Verification items for the finished model (mm, model axes). Face numbers are marked on the shaded views. A direction names the side the tool comes from. Coordinates: 2 decimals unless noted, no trailing zeros. Order: outer loops, then holes, each group sorted by start corner. A loop starts at its lowest first (then second) coordinate and runs counter-clockwise, first axis right, second up.
Q1. Cross-section at C-C, the plane y = 6.75. Record the boundary of the cut face in (x, z) (3 decimals).
Q2. Cross-section at B-B, the plane x = 6.35. Record the boundary of the cut face in (y, z).
Q3. Thickness scan on line 1 (Y direction, x = -1.27, z = 0.75); line 2 (X direction, y = 5.5, z = 2.5); line 3 (Z direction, x = -6.75, y = 10.25). Record the ranges inside material, lowest first.
Q4. Cross-section at A-A, the plane y = -3.16. Record the boundary of the cut face in (x, z).
Q5. Set-up check for the marked faces 1 and 2: record each of +Z, -Z, +X, -X, +Y, -Y from which the full face is reachable in a straight line by a thin tool's end or side.
Q6. Depth check by flat-ended pin: P1, Ø2, axis at x = 3.5, z = 3, coming from the +Y side; P2, Ø0.8, axis at x = 2, z = 3.5, coming from the +Y side; P3, Ø2, axis at x = 1, z = 3, coming from the -Y side; P4, Ø0.5, axis at y = 7, z = 2.5, coming from the -X side. Enter the tip coordinate at first touch or a pass-through.
Q7. Cross-section at D-D, the plane z = 1.25. Count the separate pieces of the cut face and the enclosed holes in it, and give its area (3 significant figures).
from build123d import *

# Parameters (mm, degrees)
SKETCH_W        = 17.7
SKETCH_H        = 21.4
PAD_DEPTH       = 1.65
SKETCH001_W     = 9
SKETCH001_H     = 7.4
PAD001_DEPTH    = 3.35
SKETCH002_R     = 0.5
POCKET_DEPTH    = 1.651
FILLET_R        = 1.675
POCKET001_DEPTH = 2
POCKET002_DEPTH = 4.5
POCKET003_DEPTH = 0.35


with BuildPart() as part:
    # Sketch → Pad (new body)
    with BuildSketch(Plane.XY):
        Rectangle(SKETCH_W, SKETCH_H)
    extrude(amount=PAD_DEPTH)

    # Sketch001 (on Face6 of Pad) → Pad001 (join)
    with BuildSketch(Plane.XY.offset(1.65)):
        with Locations((0, 7.3)):
            Rectangle(SKETCH001_W, SKETCH001_H)
    extrude(amount=PAD001_DEPTH)

    # Sketch002 (on Face5 of Pad001) → Pocket (cut, through all)
    with BuildSketch(Plane.XY.offset(1.65)):
        with Locations((-6.35, -3.16)):
            Circle(SKETCH002_R)
        with Locations((-3.81, -3.16)):
            Circle(SKETCH002_R)
        with Locations((-1.27, -3.16)):
            Circle(SKETCH002_R)
        with Locations((1.27, -3.16)):
            Circle(SKETCH002_R)
        with Locations((3.81, -3.16)):
            Circle(SKETCH002_R)
        with Locations((6.35, -3.16)):
            Circle(SKETCH002_R)
        with Locations((-6.35, -5.7)):
            Circle(SKETCH002_R)
        with Locations((-3.81, -5.7)):
            Circle(SKETCH002_R)
        with Locations((-1.27, -5.7)):
            Circle(SKETCH002_R)
        with Locations((1.27, -5.7)):
            Circle(SKETCH002_R)
        with Locations((3.81, -5.7)):
            Circle(SKETCH002_R)
        with Locations((6.35, -5.7)):
            Circle(SKETCH002_R)
    extrude(amount=-POCKET_DEPTH, mode=Mode.SUBTRACT)

    # Fillet
    fillet_edges = [part.edges().sort_by_distance(p)[0] for p in [
        (-4.5, 7.3, 5),
        (4.5, 7.3, 5),
    ]]
    fillet(fillet_edges, radius=FILLET_R)

    # Sketch003 (on Face5 of Fillet) → Pocket001 (cut)
    with BuildSketch(Plane(origin=(0, 11, 0), x_dir=(-1, 0, 0), z_dir=(0, 1, 0))):
        with BuildLine():
            ThreePointArc((-4.5, 3.325), (-4.009404, 2.140596), (-2.825, 1.65))
            Line((-2.825, 1.65), (-4.5, 1.65))
            Line((-4.5, 3.325), (-4.5, 1.65))
        make_face()
        with BuildLine():
            ThreePointArc((2.825, 1.65), (4.009404, 2.140596), (4.5, 3.325))
            Line((4.5, 3.325), (4.5, 1.65))
            Line((2.825, 1.65), (4.5, 1.65))
        make_face()
    extrude(amount=-POCKET001_DEPTH, mode=Mode.SUBTRACT)

    # Sketch004 (on Face6 of Pocket001) → Pocket002 (cut)
    with BuildSketch(Plane(origin=(0, 11, 0), x_dir=(-1, 0, 0), z_dir=(0, 1, 0))):
        with BuildLine():
            ThreePointArc((-2.825, 4.7), (-4.2, 3.325), (-2.825, 1.95))
            Line((-2.825, 1.95), (2.825, 1.95))
            ThreePointArc((2.825, 1.95), (4.2, 3.325), (2.825, 4.7))
            Line((2.825, 4.7), (-2.825, 4.7))
        make_face()
        with BuildLine():
            ThreePointArc((-2.825, 3.65), (-3.15, 3.325), (-2.825, 3))
            Line((-2.825, 3), (2.825, 3))
            ThreePointArc((2.825, 3), (3.15, 3.325), (2.825, 3.65))
            Line((2.825, 3.65), (-2.825, 3.65))
        make_face(mode=Mode.SUBTRACT)
    extrude(amount=-POCKET002_DEPTH, mode=Mode.SUBTRACT)

    # Pocket002 Face38 → Pocket003 (cut)
    with BuildSketch(Plane(origin=(0, 11, 3.325), x_dir=(1, 0, 0), z_dir=(0, 1, 0))):
        with BuildLine():
            Line((-2.825, -0.325), (2.825, -0.325))
            ThreePointArc((2.825, -0.325), (3.15, 0), (2.825, 0.325))
            Line((2.825, 0.325), (-2.825, 0.325))
            ThreePointArc((-2.825, 0.325), (-3.15, 0), (-2.825, -0.325))
        make_face()
    extrude(amount=-POCKET003_DEPTH, mode=Mode.SUBTRACT)


solid = part.part
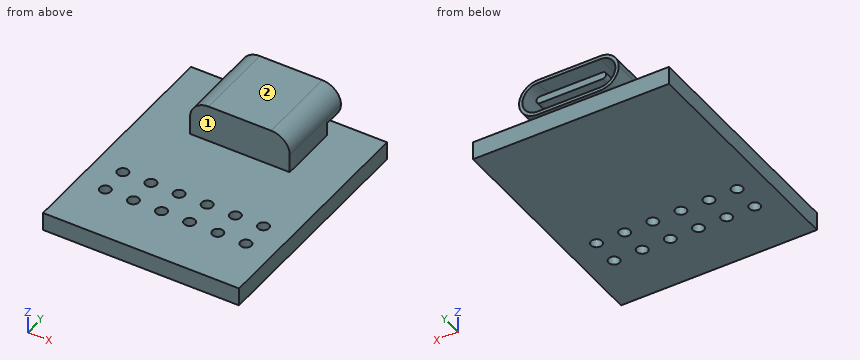
Check values:
1. outline: (-8.85, 0) - (8.85, 0) - (8.85, 1.65) - (4.5, 1.65) - (4.5, 3.325) arc R1.675 ccw to (2.825, 5) - (-2.825, 5) arc R1.675 ccw to (-4.5, 3.325) - (-4.5, 1.65) - (-8.85, 1.65) - close; (-2.825, 3) - (2.825, 3) arc R0.325 ccw to (2.825, 3.65) - (-2.825, 3.65) arc R0.325 ccw to start; hole (-2.825, 1.95) - (2.825, 1.95) arc R1.375 ccw to (2.825, 4.7) - (-2.825, 4.7) arc R1.375 ccw to start
2. outline: (-10.7, 0) - (-6.2, 0) - (-6.2, 1.65) - (-10.7, 1.65) - close; (-5.2, 0) - (-3.66, 0) - (-3.66, 1.65) - (-5.2, 1.65) - close; (-2.66, 0) - (10.7, 0) - (10.7, 1.65) - (-2.66, 1.65) - close
3. line 1: y = -10.7 to -6.2, -5.2 to -3.66, -2.66 to 10.7
3. line 2: x = -4.5 to 4.5
3. line 3: z = 0 to 1.65
4. outline: (-8.85, 0) - (-6.85, 0) - (-6.85, 1.65) - (-8.85, 1.65) - close; (-5.85, 0) - (-4.31, 0) - (-4.31, 1.65) - (-5.85, 1.65) - close; (-3.31, 0) - (-1.77, 0) - (-1.77, 1.65) - (-3.31, 1.65) - close; (-0.77, 0) - (0.77, 0) - (0.77, 1.65) - (-0.77, 1.65) - close; (1.77, 0) - (3.31, 0) - (3.31, 1.65) - (1.77, 1.65) - close; (4.31, 0) - (5.85, 0) - (5.85, 1.65) - (4.31, 1.65) - close; (6.85, 0) - (8.85, 0) - (8.85, 1.65) - (6.85, 1.65) - close
5. face 1: +Z, +X, -X, -Y
5. face 2: +Z, +X, -X, +Y, -Y
6. P1: stops at y = 11
6. P2: stops at y = 10.65
6. P3: stops at y = 3.6
6. P4: stops at x = -4.5
7. separate pieces: 1
7. enclosed holes: 12
7. area: 369 mm2
